Geometry: final body of the model. Coordinates: model frame, mm. Give positions to 0.01 mm unless a question says otherwise; leave off trailing zeros. Write each loop counter-clockwise with the first axis right and the second up, starting at its lowest first coordinate (ties: lowest second). Pieces come first, ordered by that corner, then holes. Notation, with made-up numbers: (31, 35.25) -> (78, 35.25) arc R21 ccw to (78, 67.25) -> close; hole circle Ø3 at (86, 52). An arc over 180 degrees is marked (long way). Answer in a Markdown table with one row per item. Add a question column.
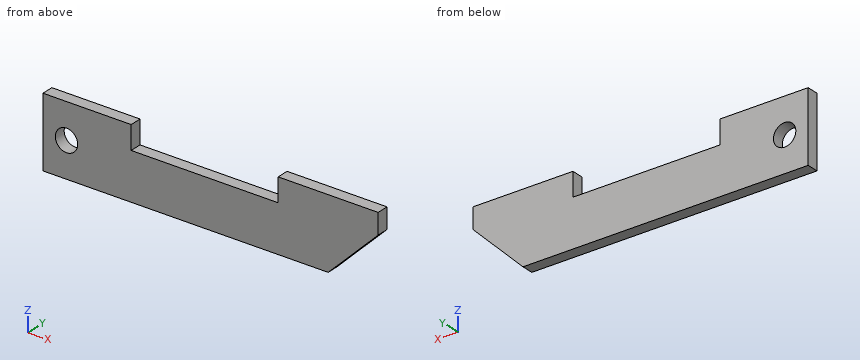
from build123d import *

# Parameters (mm, degrees)
SKETCH_1_R      = 1.9
EXTRUDE_1_DEPTH = 2


with BuildPart() as part:
    # Эскиз1 → Бобышка-Вытянуть1 (new body)
    with BuildSketch(Plane(origin=(0, 0, 0), x_dir=(1, 0, 0), z_dir=(0, 1, 0))):
        Polygon((0, 0), (48.5, 0), (57, -8.5), (57, -12), (40, -12), (40, -8), (15, -8), (15, -12), (0, -12), align=None)
        with Locations((4, -6)):
            Circle(SKETCH_1_R, mode=Mode.SUBTRACT)
    extrude(amount=EXTRUDE_1_DEPTH)


solid = part.part
Q1. Section A-A on z = 10. Return loops of the section in (x, y), and give its area (3 significant figures).
Q2. Section C-C on x = 4. Return loops of the section in (y, z), and give its area (3 significant figures).
Q3. Section B-B on y = 1.5. Return loops of the section in (x, z).
Q4. Section D-D on x = 34. Return loops of the section in (y, z), and give its area (3 significant figures).
Q5. Line query: probe 1 along X at (y, z) = (1.95, 8.75); probe 2 along Z at (x, y) = (4, 0.9); probe 3 along Z at (x, y) = (21, 0.15). Output: solid intervals per line, ascending. Write a range as from..to.
Checks:
| question | item | result |
|---|---|---|
| 1 | outline | (0, 0) -> (15, 0) -> (15, 2) -> (0, 2) -> close; (40, 0) -> (57, 0) -> (57, 2) -> (40, 2) -> close |
| 1 | area | 64.0 mm^2 |
| 2 | outline | (0, 0) -> (2, 0) -> (2, 4.1) -> (0, 4.1) -> close; (0, 7.9) -> (2, 7.9) -> (2, 12) -> (0, 12) -> close |
| 2 | area | 16.4 mm^2 |
| 3 | outline | (0, 0) -> (48.5, 0) -> (57, 8.5) -> (57, 12) -> (40, 12) -> (40, 8) -> (15, 8) -> (15, 12) -> (0, 12) -> close; hole circle Ø3.8 at (4, 6) |
| 4 | outline | (0, 0) -> (2, 0) -> (2, 8) -> (0, 8) -> close |
| 4 | area | 16.0 mm^2 |
| 5 | probe 1 | 0..15, 40..57 |
| 5 | probe 2 | 0..4.1, 7.9..12 |
| 5 | probe 3 | 0..8 |
